The model under review builds one solid part; all positions refer to its coordinate system, in mm. A direction names the side the tool comes from. Coordinates: 2 decimals unless noted, no trailing zeros. Loops run counter-clockwise (first coordinate to the right, second up) from the corner with the lowest first, then second, coordinate; pieces in that order, holes last. Notation, with made-up numbers: M 80,12.25 L 139,12.25 A32 ccw 139,41.25 Z; hole C 25.5,89.5 d7. An arc over 180 degrees is marked long. Return JSON: item names as keys, results as strings.
```python
from build123d import *

# Parameters (mm, degrees)
SKETCH1_W          = 2200
SKETCH1_H          = 1100
EXTRUDE1_DEPTH     = 1050
SHELL1_T           = -10
SKETCH2_W          = 600
SKETCH2_H          = 600
CUT_EXTRUDE1_DEPTH = 400


with BuildPart() as part:
    # Sketch1 → Extrude1 (new body)
    with BuildSketch(Plane(origin=(0, 0, 0), x_dir=(1, 0, 0), z_dir=(0, 1, 0))):
        with Locations((-1100, 550)):
            Rectangle(SKETCH1_W, SKETCH1_H)
    extrude(amount=EXTRUDE1_DEPTH)

    # Shell1
    shell1_openings = [part.faces().sort_by_distance(p)[0] for p in [
        (-1100, 1050, -550),
    ]]
    offset(amount=SHELL1_T, openings=shell1_openings, kind=Kind.INTERSECTION)

    # Sketch2 → Cut-Extrude1 (cut)
    with BuildSketch(Plane.XZ):
        with Locations((-400, -550)):
            Rectangle(SKETCH2_W, SKETCH2_H)
    extrude(amount=-CUT_EXTRUDE1_DEPTH, mode=Mode.SUBTRACT)


solid = part.part
```
1. The part is to be moulded in two halves that separate along Z. For faces 1 (the face through (-10, 523, -542)), 2 (the face through (-1360, 0, -558)), 3 (the face through (-1115, 518, -1100)), say which applies: released by +Z, released by -Z, zero draft, split by the parting line, or undercut.
Check values:
{"face 1": "undercut", "face 2": "zero draft", "face 3": "released by -Z"}
2. Machinability: for faces 4 (the face through (-1115, 523, -10)), 5 (the face through (-1115, 518, 0)), which of the approach directions +Z, -Z, +X, -X, +Y, -Y give a long, thin tool a straight path to every point of the face, cutting with its end or side? Answer none if there is none.
Check values:
{"face 4": "+Y", "face 5": "+Z, +X, -X, +Y, -Y"}
3. Add section C-C on z = -809. Give the boundary of the cut face in (x, y).
Check values:
{"outline": "M -2200,0 L -700,0 L -700,10 L -2190,10 L -2190,1050 L -2200,1050 Z; M -100,0 L 0,0 L 0,1050 L -10,1050 L -10,10 L -100,10 Z"}
4. Add section B-B on y = 395. Give the boundary of the cut face in (x, z), plus the area to 3 significant figures.
Check values:
{"outline": "M -2200,-1100 L 0,-1100 L 0,0 L -2200,0 Z; hole M -2190,-1090 L -10,-1090 L -10,-10 L -2190,-10 Z", "area": "65,600 mm²"}
5. Add section A-A on x = -481. Give the boundary of the cut face in (y, z), plus the area to 3 significant figures.
Check values:
{"outline": "M 0,-1100 L 1050,-1100 L 1050,-1090 L 10,-1090 L 10,-850 L 0,-850 Z; M 0,-250 L 10,-250 L 10,-10 L 1050,-10 L 1050,0 L 0,0 Z", "area": "25,800 mm²"}
6. Add section D-D on z = -212.5. Give the boundary of the cut face in (x, y).
Check values:
{"outline": "M -2200,0 L 0,0 L 0,1050 L -10,1050 L -10,10 L -2190,10 L -2190,1050 L -2200,1050 Z"}
7. To check wall thickness, follow line 1 (X direction, y = 781, z = -749.5); line 2 (Z direction, x = -548, y = 604); line 3 (Y direction, x = -1068, z = -865). State the ranges of each line that lie inside material, in increasing order.
Check values:
{"line 1": "-2200 to -2190, -10 to 0", "line 2": "-1100 to -1090, -10 to 0", "line 3": "0 to 10"}
